Read the model definition and answer for the solid it produces. Units are mm, in the model's axes. A direction names the side the tool comes from. Coordinates: 2 decimals unless noted, no trailing zeros. Loops run counter-clockwise (first coordinate to the right, second up) from the corner with the lowest first, then second, coordinate; pieces in that order, holes last. Notation, with made-up numbers: (24, 48.25) -> (68, 48.25) arc R12 ccw to (68, 64.25) -> close; hole circle Ø9 at (-1, 77). An arc over 180 degrees is marked (long way). Answer as a JSON object with one key per item and string values. Group by question number.
1) Determine the mould class of faces 1 (the face through (60, 22, 7)), 2 (the face through (30, 41, 5.15)), 3 (the face through (23, 8, 0)) for opening direction X: released by +X, released by -X, zero draft, split by the parting line, or undercut.
2) Which of the six approach directions +Z, -Z, +X, -X, +Y, -Y give full straight-line access (tool end or side, diameter ignored) to faces 4 (the face through (57.95, 35, 10)), 5 (the face through (58.247, 4.393, 4.437)), 6 (the face through (30, 9.9, 3))?
3) Consider probe 1 along Y at (x, z) = (55, 4.75); probe 2 along Y at (x, z) = (5, 11.2); probe 3 along Y at (x, z) = (5, 10.3). Determine where each line is inside the solid, lowest interval first. Write a range as [from, to].
4) Section C-C, the plane z = 12.75 is taken. Count the separate pieces of the cut face and the enclosed holes in it, plus the area to 3 significant figures.
5) Flat-ended cylindrical pins translate along their axes: P1, Ø6, axis at x = 47.5, y = 35.5, coming from the +Z side; P2, Ø2, axis at x = 4.5, y = 42, coming from the -Z side; P3, Ø6, axis at x = 24, z = 11, coming from the +Y side. Find the tip coordinate at first contact, or state that the pin passes through.
6) Section B-B, the plane x = 55 is taken. Give the vertices of the cut face in (y, z).
7) Section A-A, the plane z = 7.25 is taken. Give the vertices of the cut face in (x, y).
8) Section D-D, the plane x = 32.5 is taken. Give the vertices of the cut face in (y, z).
Autodesk Inventor part; units mm, degrees
ref_plane "YZ Plane" through (0, 0, 0) normal (1, 0, 0) x (0, 1, 0)
ref_plane "XZ Plane" through (0, 0, 0) normal (0, 1, 0) x (-1, 0, 0)
ref_plane "XY Plane" through (0, 0, 0) normal (0, 0, 1) x (1, 0, 0)
sketch "Sketch2" plane through (0, 0, 0) normal (0, 0, 1) x (1, 0, 0)
  line L0 (0, 0) -> (60, 0)
  line L1 (60, 0) -> (60, 45)
  line L2 (60, 45) -> (0, 45)
  line L3 (0, 45) -> (0, 0)
  dimension "d0" = 60
  dimension "d1" = 45
extrude "Cover_Body" add sketch "Sketch2" along normal blind 15
sketch "Sketch4" plane through (0, 0, 15) normal (0, 0, 1) x (1, 0, 0)
  line L0 (60, 45) -> (0, 45)
  line L1 (0, 45) -> (0, 0)
  line L2 (2.75, 33.35) -> (10.45, 33.35)
  line L3 (50.25, 33.35) -> (57.95, 33.35)
  line L4 (60, 0) -> (60, 45)
  line L5 (0, 0) -> (60, 0)
  line L6 (2.75, 33.35) -> (2.75, 36.65)
  line L7 (2.75, 36.65) -> (10.45, 36.65)
  line L8 (10.45, 36.65) -> (10.45, 45)
  line L9 (57.95, 36.65) -> (57.95, 33.35)
  line L10 (57.95, 36.65) -> (50.25, 36.65)
  line L11 (50.25, 36.65) -> (50.25, 45)
  line L12 (10.45, 45) -> (50.25, 45)
  line L13 (30, 36.5125) -> (30, -47.625) construction
  line L14 (50.25, 33.35) -> (50.25, 0)
  line L15 (10.45, 33.35) -> (10.45, 0)
  line L16 (10.45, 0) -> (50.25, 0)
  line L17 (-12.9814, 35) -> (83.563, 35) construction
  dimension "d6" = 7.7
  dimension "d14" = 3.3
  dimension "d15" = 3.3
  dimension "d22" = 60
  dimension "d23" = 30
  dimension "d28" = 7.7
  dimension "d118" = 39.8
  dimension "d130" = 33.35
  dimension "d140" = 36.65
  dimension "d141" = 10
  dimension "d142" = 10.45
extrude "Servo_Intake" cut sketch "Sketch4" against normal blind 9.85 contours L11 L10 L9 L3 L14 L5 L15 L2 L6 L7 L8 L0
sketch "Sketch5" plane through (0, 0, 15) normal (0, 0, 1) x (1, 0, 0)
  line L0 (0, 5.9) -> (0, 8.9)
  line L1 (-28.5301, 7.4) -> (55.9395, 7.4) construction
  line L2 (0, 8.9) -> (10.45, 8.9)
  line L3 (10.45, 8.9) -> (10.45, 5.9)
  line L4 (10.45, 5.9) -> (0, 5.9)
  line L5 (10.45, 0) -> (10.45, 33.35)
  line L6 (0, 45) -> (0, 0)
  line L7 (0, 0) -> (10.45, 0)
  dimension "d97" = 3
  dimension "d137" = 5.9
  dimension "d153" = 7.4
extrude "Cable_Opening" cut sketch "Sketch5" against normal blind 4 contours L0 L2 L3 L4
sketch "Sketch6" plane through (0, 0, 15) normal (0, 0, 1) x (1, 0, 0)
  circle A0 centre (5, 40.75) radius 1.7
  circle A1 centre (55, 40.75) radius 1.7
  circle A2 centre (55, 4.25) radius 1.7
  circle A3 centre (5, 4.25) radius 1.7
  line L0 (30, 47.1) -> (30, -0.525) construction
  line L1 (-11.6375, 22.5) -> (75.675, 22.5) construction
  line L2 (60, 0) -> (60, 45)
  line L3 (0, 45) -> (0, 0)
  line L4 (10.45, 45) -> (0, 45)
  line L5 (0, 0) -> (60, 0)
  point P0 (42, 12.35)
  point P1 (0, 12.35)
  dimension "d29" = 3.4
  dimension "d30" = 3.4
  dimension "d31" = 3.4
  dimension "d32" = 3.4
  dimension "d33" = 60
  dimension "d34" = 30
  dimension "d35" = 45
  dimension "d36" = 22.5
  dimension "d37" = 50
  dimension "d38" = 25
  dimension "d39" = 36.5
  dimension "d40" = 18.25
extrude "Screw_Holes" cut sketch "Sketch6" against normal blind 36.5
sketch "Sketch16" plane through (0, 0, 0) normal (0, 0, -1) x (-1, 0, 0)
  circle A0 centre (-55, 4.25) radius 3.25
  circle A1 centre (-5, 40.75) radius 3.25
  circle A2 centre (-55, 4.25) radius 1.7
  circle A3 centre (-5, 40.75) radius 1.7
  circle A4 centre (-5, 4.25) radius 1.7
  circle A5 centre (-5, 4.25) radius 3.25
  circle A6 centre (-55, 40.75) radius 1.7
  circle A7 centre (-55, 40.75) radius 3.25
  dimension "d99" = 6.5
  dimension "d100" = 6.5
  dimension "d151" = 6.5
  dimension "d152" = 6.5
extrude "Screw_Pockets" cut sketch "Sketch16" against normal blind 9 contours A0 | A1 | A2 | A3 | A5 | A7
sketch "Sketch24" plane through (0, 0, 5.15) normal (0, 0, 1) x (1, 0, 0)
  line L0 (10.45, 9.9) -> (50.25, 9.9)
  line L1 (50.25, 9.9) -> (50.25, 40)
  line L2 (50.25, 40) -> (10.45, 40)
  line L3 (10.45, 40) -> (10.45, 9.9)
  line L4 (50.25, 0) -> (10.45, 0)
  line L5 (10.45, 45) -> (50.25, 45)
  line L6 (10.45, 0) -> (10.45, 33.35)
  line L7 (50.25, 33.35) -> (50.25, 0)
  point P0 (0, 0)
  dimension "d143" = 9.9
  dimension "d144" = 5
extrude "Cooling_Opening" cut sketch "Sketch24" against normal up to surface (5.15 mm away) contours L3 L2 L1 L0
chamfer "Chamfer1" distance 2 angle 45 4 edges at (10.45, 9.9, 2.575) (50.25, 9.9, 2.575) (50.25, 40, 2.575) (10.45, 40, 2.575)
fillet "Fillet2" radius 2 4 edges at (10.45, 36.65, 10.075) (10.45, 33.35, 10.075) (50.25, 36.65, 10.075) (50.25, 33.35, 10.075)
equation "\"d15\" = d14"
equation "\"d23\" = 0.5 * d22"
equation "\"d28\" = d6"
equation "\"d30\" = d29"
equation "\"d31\" = d29"
equation "\"d32\" = d29"
equation "\"d34\" = 0.5 * d33"
equation "\"d36\" = 0.5 * d35"
equation "\"d38\" = 0.5 * d37"
equation "\"d40\" = 0.5 * d39"
equation "\"d41\" = d39"
equation "\"d99\" = d100"
equation "\"d151\" = d100"
equation "\"d152\" = d100"
properties part number "EDMO1-1_Cover" material "PLA"
Determined:
{
 "1": {"face 1": "released by +X", "face 2": "undercut", "face 3": "zero draft"},
 "2": {"face 4": "+Z", "face 5": "-Z", "face 6": "+Z, -Z"},
 "3": {"probe 1": "[0, 1], [7.5, 37.5], [44, 45]", "probe 2": "[0, 2.55], [8.9, 33.35], [36.65, 39.05], [42.45, 45]", "probe 3": "[0, 2.55], [5.95, 33.35], [36.65, 39.05], [42.45, 45]"},
 "4": {"separate pieces": "3", "enclosed holes": "3", "area": "787 mm²"},
 "5": {"P1": "z = 5.15", "P2": "z = 9", "P3": "through"},
 "6": {"outline": "(0, 0) -> (1, 0) -> (1, 9) -> (2.55, 9) -> (2.55, 15) -> (0, 15) -> close; (5.95, 9) -> (7.5, 9) -> (7.5, 0) -> (37.5, 0) -> (37.5, 9) -> (39.05, 9) -> (39.05, 15) -> (36.65, 15) -> (36.65, 5.15) -> (33.35, 5.15) -> (33.35, 15) -> (5.95, 15) -> close; (42.45, 9) -> (44, 9) -> (44, 0) -> (45, 0) -> (45, 15) -> (42.45, 15) -> close"},
 "7": {"outline": "(0, 0) -> (10.45, 0) -> (10.45, 31.35) arc R2 ccw to (8.45, 33.35) -> (2.75, 33.35) -> (2.75, 36.65) -> (8.45, 36.65) arc R2 ccw to (10.45, 38.65) -> (10.45, 45) -> (0, 45) -> close; (50.25, 0) -> (60, 0) -> (60, 45) -> (50.25, 45) -> (50.25, 38.65) arc R2 ccw to (52.25, 36.65) -> (57.95, 36.65) -> (57.95, 33.35) -> (52.25, 33.35) arc R2 ccw to (50.25, 31.35) -> close; hole circle Ø6.5 at (5, 4.25); hole circle Ø6.5 at (5, 40.75); hole circle Ø6.5 at (55, 4.25); hole circle Ø6.5 at (55, 40.75)"},
 "8": {"outline": "(0, 0) -> (9.9, 0) -> (9.9, 5.15) -> (0, 5.15) -> close; (40, 0) -> (45, 0) -> (45, 5.15) -> (40, 5.15) -> close"}
}
